```python
from build123d import *

# Parameters (mm, degrees)
MAIN_SHAPE_DEPTH        = 0.6
TABS_DEPTH              = 154.060061459
TABS_DEPTH_BACK         = 154.060061459
CHIN_GUARD_DEPTH        = 0.6
FILLET1_R               = 30
SKETCH8_W               = 100
SKETCH8_H               = 1
CUT_EXTRUDE3_DEPTH      = 0.2
BOSS_EXTRUDE1_START     = -0.6
BOSS_EXTRUDE1_DEPTH     = 0.6
CUT_EXTRUDE4_DEPTH      = 173.475044334
CUT_EXTRUDE4_DEPTH_BACK = 173.475044334
FILLET2_R               = 0.5
FILLET3_R               = 1.5


with BuildPart() as part:
    # Sketch1 → Main Shape (new body)
    with BuildSketch(Plane.XY):
        with BuildLine():
            Line((-24, -91.764766734), (24, -91.764766734))
            Line((24, -91.764766734), (78.266232563, -84.05670244))
            ThreePointArc((78.266232563, -84.05670244), (97.655491519, -79.289252293), (115.711102551, -70.764766734))
            ThreePointArc((115.711102551, -70.764766734), (120.685143325, -65.658407438), (122.5, -58.764766734))
            ThreePointArc((122.5, -58.764766734), (120.227482046, -43.118277124), (113.597722286, -28.764766734))
            ThreePointArc((113.597722286, -28.764766734), (107.811505455, -22.955172168), (100.180351554, -19.955641477))
            Line((100.180351554, -19.955641477), (60.74391922, -13.264766734))
            ThreePointArc((60.74391922, -13.264766734), (50.804108255, -9.246591688), (43.461443341, -1.434367632))
            ThreePointArc((43.461443341, -1.434367632), (36.448172688, 5.805997675), (26.941855461, 9.15842781))
            Line((26.941855461, 9.15842781), (17, 10.235233266))
            Line((17, 10.235233266), (10, 0))
            Line((10, 0), (-10, 0))
            Line((-10, 0), (-17, 10.235233266))
            Line((-17, 10.235233266), (-26.941855461, 9.15842781))
            ThreePointArc((-26.941855461, 9.15842781), (-36.448172688, 5.805997675), (-43.461443341, -1.434367632))
            ThreePointArc((-43.461443341, -1.434367632), (-50.804108255, -9.246591688), (-60.74391922, -13.264766734))
            Line((-60.74391922, -13.264766734), (-100.180351554, -19.955641477))
            ThreePointArc((-100.180351554, -19.955641477), (-107.811505455, -22.955172168), (-113.597722286, -28.764766734))
            ThreePointArc((-113.597722286, -28.764766734), (-120.227482046, -43.118277124), (-122.5, -58.764766734))
            ThreePointArc((-122.5, -58.764766734), (-120.685143325, -65.658407438), (-115.711102551, -70.764766734))
            ThreePointArc((-115.711102551, -70.764766734), (-97.655491519, -79.289252293), (-78.266232563, -84.05670244))
            Line((-78.266232563, -84.05670244), (-24, -91.764766734))
        make_face()
    extrude(amount=MAIN_SHAPE_DEPTH)

    # Sketch2 → Tabs (cut, two sides: drawn at the far end of the back side and taken through both)
    with BuildSketch(Plane.XY.offset(0.6).offset(-TABS_DEPTH_BACK)):
        with BuildLine():
            Line((-121.15, -59.764766734), (-121.15, -57.764766734))
            Line((-121.15, -57.764766734), (-115.985504489, -54.767473344))
            ThreePointArc((-115.985504489, -54.767473344), (-113.65344245, -43.380285918), (-108.686779625, -32.871298753))
            Line((-108.686779625, -32.871298753), (-111.02, -27.374766734))
            Line((-111.02, -27.374766734), (-109.82, -25.774766734))
            Line((-109.82, -25.774766734), (-107.82, -24.774766734))
            Line((-107.82, -24.774766734), (-106.22, -25.974766734))
            Line((-106.22, -25.974766734), (-107.42, -27.574766734))
            Line((-107.42, -27.574766734), (-105.82, -28.774766734))
            Line((-105.82, -28.774766734), (-99.063546264, -19.766161753))
            Line((-99.063546264, -19.766161753), (-100.180351554, -19.955641477))
            ThreePointArc((-100.180351554, -19.955641477), (-107.811505455, -22.955172168), (-113.597722286, -28.764766734))
            ThreePointArc((-113.597722286, -28.764766734), (-120.227482046, -43.118277124), (-122.5, -58.764766734))
            ThreePointArc((-122.5, -58.764766734), (-120.810564569, -65.431850055), (-116.15, -70.489846692))
            Line((-116.15, -70.489846692), (-116.15, -59.764766734))
            Line((-116.15, -59.764766734), (-118.15, -59.764766734))
            Line((-118.15, -59.764766734), (-118.15, -61.764766734))
            Line((-118.15, -61.764766734), (-120.15, -61.764766734))
            Line((-120.15, -61.764766734), (-121.15, -59.764766734))
        make_face()
        with BuildLine():
            Line((105.82, -28.774766734), (99.063546264, -19.766161753))
            Line((99.063546264, -19.766161753), (100.180351554, -19.955641477))
            ThreePointArc((100.180351554, -19.955641477), (107.811505455, -22.955172168), (113.597722286, -28.764766734))
            ThreePointArc((113.597722286, -28.764766734), (120.227482046, -43.118277124), (122.5, -58.764766734))
            ThreePointArc((122.5, -58.764766734), (120.810564569, -65.431850055), (116.15, -70.489846692))
            Line((116.15, -70.489846692), (116.15, -59.764766734))
            Line((116.15, -59.764766734), (118.15, -59.764766734))
            Line((118.15, -59.764766734), (118.15, -61.764766734))
            Line((118.15, -61.764766734), (120.15, -61.764766734))
            Line((120.15, -61.764766734), (121.15, -59.764766734))
            Line((121.15, -59.764766734), (121.15, -57.764766734))
            Line((121.15, -57.764766734), (115.985504489, -54.767473344))
            ThreePointArc((115.985504489, -54.767473344), (113.65344245, -43.380285918), (108.686779625, -32.871298753))
            Line((108.686779625, -32.871298753), (111.02, -27.374766734))
            Line((111.02, -27.374766734), (109.82, -25.774766734))
            Line((109.82, -25.774766734), (107.82, -24.774766734))
            Line((107.82, -24.774766734), (106.22, -25.974766734))
            Line((106.22, -25.974766734), (107.42, -27.574766734))
            Line((107.42, -27.574766734), (105.82, -28.774766734))
        make_face()
    extrude(amount=TABS_DEPTH + TABS_DEPTH_BACK, mode=Mode.SUBTRACT)

    # Sketch5 → Chin guard (add)
    with BuildSketch(Plane.XY.offset(0.6)):
        Polygon((-78.266232563, -84.05670244), (-24, -121.764766734), (24, -121.764766734), (78.266232563, -84.05670244), (24, -91.764766734), (-24, -91.764766734), align=None)
    extrude(amount=-CHIN_GUARD_DEPTH)

    # Fillet1
    fillet1_edges = [part.edges().sort_by_distance(p)[0] for p in [
        (-24, -121.764766734, 0.3),
        (24, -121.764766734, 0.3),
        (78.266232563, -84.05670244, 0.3),
        (-78.266232563, -84.05670244, 0.3),
    ]]
    fillet(fillet1_edges, radius=FILLET1_R)

    # Sketch8 → Cut-Extrude3 (cut)
    with BuildSketch(Plane.XY.offset(0.6)):
        with Locations((0, -4.5)):
            Rectangle(SKETCH8_W, SKETCH8_H)
    extrude(amount=-CUT_EXTRUDE3_DEPTH, mode=Mode.SUBTRACT)

    # Sketch9 → Boss-Extrude1 (add)
    with BuildSketch(Plane.XY.offset(0.6).offset(BOSS_EXTRUDE1_START)):
        with BuildLine():
            Line((-121.15, -61.764766734), (-120.15, -61.764766734))
            Line((-120.15, -61.764766734), (-121.15, -59.764766734))
            Line((-121.15, -59.764766734), (-121.15, -57.764766734))
            Line((-121.15, -57.764766734), (-115.985504489, -54.767473344))
            ThreePointArc((-115.985504489, -54.767473344), (-115.959300984, -54.461436848), (-115.931165822, -54.155571889))
            Line((-115.931165822, -54.155571889), (-122.15, -57.764766734))
            Line((-122.15, -57.764766734), (-122.15, -59.764766734))
            Line((-122.15, -59.764766734), (-121.15, -61.764766734))
        make_face()
        with BuildLine():
            Line((-111.02, -27.374766734), (-108.686779625, -32.871298753))
            ThreePointArc((-108.686779625, -32.871298753), (-108.849438719, -33.131850053), (-109.010449565, -33.393423117))
            Line((-109.010449565, -33.393423117), (-111.82, -26.774766734))
            Line((-111.82, -26.774766734), (-110.62, -25.174766734))
            Line((-110.62, -25.174766734), (-108.62, -24.174766734))
            Line((-108.62, -24.174766734), (-107.82, -24.774766734))
            Line((-107.82, -24.774766734), (-109.82, -25.774766734))
            Line((-109.82, -25.774766734), (-111.02, -27.374766734))
        make_face()
        with BuildLine():
            Line((108.62, -24.174766734), (107.82, -24.774766734))
            Line((107.82, -24.774766734), (109.82, -25.774766734))
            Line((109.82, -25.774766734), (111.02, -27.374766734))
            Line((111.02, -27.374766734), (108.686779625, -32.871298753))
            ThreePointArc((108.686779625, -32.871298753), (108.849438719, -33.131850053), (109.010449565, -33.393423117))
            Line((109.010449565, -33.393423117), (111.82, -26.774766734))
            Line((111.82, -26.774766734), (110.62, -25.174766734))
            Line((110.62, -25.174766734), (108.62, -24.174766734))
        make_face()
        with BuildLine():
            Line((121.15, -57.764766734), (115.985504489, -54.767473344))
            ThreePointArc((115.985504489, -54.767473344), (115.959300984, -54.461436848), (115.931165822, -54.155571889))
            Line((115.931165822, -54.155571889), (122.15, -57.764766734))
            Line((122.15, -57.764766734), (122.15, -59.764766734))
            Line((122.15, -59.764766734), (121.15, -61.764766734))
            Line((121.15, -61.764766734), (120.15, -61.764766734))
            Line((120.15, -61.764766734), (121.15, -59.764766734))
            Line((121.15, -59.764766734), (121.15, -57.764766734))
        make_face()
    extrude(amount=BOSS_EXTRUDE1_DEPTH)

    # Sketch7 → Cut-Extrude4 (cut, two sides: drawn at the far end of the back side and taken through both)
    with BuildSketch(Plane.XY.offset(0.6).offset(-CUT_EXTRUDE4_DEPTH_BACK)):
        with BuildLine():
            Line((-103.838644773, -41.913383247), (-112.792739682, -41.005537243))
            ThreePointArc((-112.792739682, -41.005537243), (-111.068159087, -37.116718005), (-109.010449565, -33.393423117))
            Line((-109.010449565, -33.393423117), (-102.436901217, -38.323584378))
            ThreePointArc((-102.436901217, -38.323584378), (-101.773894786, -40.651050555), (-103.838644773, -41.913383247))
        make_face()
        with BuildLine():
            Line((109.010449565, -33.393423117), (102.436901217, -38.323584378))
            ThreePointArc((102.436901217, -38.323584378), (101.773894786, -40.651050555), (103.838644773, -41.913383247))
            Line((103.838644773, -41.913383247), (112.792739682, -41.005537243))
            ThreePointArc((112.792739682, -41.005537243), (111.068159087, -37.116718005), (109.010449565, -33.393423117))
        make_face()
    extrude(amount=CUT_EXTRUDE4_DEPTH + CUT_EXTRUDE4_DEPTH_BACK, mode=Mode.SUBTRACT)

    # Fillet2
    fillet2_edges = [part.edges().sort_by_distance(p)[0] for p in [
        (109.010449565, -33.393423117, 0.3),
        (-112.792739682, -41.005537243, 0.3),
        (-109.010449565, -33.393423117, 0.3),
        (-106.22, -25.974766734, 0.3),
        (-107.42, -27.574766734, 0.3),
        (-105.82, -28.774766734, 0.3),
        (-115.931165822, -54.155571889, 0.3),
        (-118.15, -61.764766734, 0.3),
        (-116.15, -59.764766734, 0.3),
        (-118.15, -59.764766734, 0.3),
        (118.15, -61.764766734, 0.3),
        (118.15, -59.764766734, 0.3),
        (116.15, -59.764766734, 0.3),
        (105.82, -28.774766734, 0.3),
        (107.42, -27.574766734, 0.3),
        (106.22, -25.974766734, 0.3),
        (116.15, -70.489846692, 0.3),
        (115.931165822, -54.155571889, 0.3),
        (112.792739682, -41.005537243, 0.3),
        (99.063546264, -19.766161753, 0.3),
        (-99.063546264, -19.766161753, 0.3),
        (-116.15, -70.489846692, 0.3),
    ]]
    fillet(fillet2_edges, radius=FILLET2_R)

    # Fillet3
    fillet3_edges = [part.edges().sort_by_distance(p)[0] for p in [
        (-122.15, -57.764766734, 0.3),
        (-122.15, -59.764766734, 0.3),
        (-121.15, -61.764766734, 0.3),
        (-108.62, -24.174766734, 0.3),
        (-110.62, -25.174766734, 0.3),
        (-111.82, -26.774766734, 0.3),
        (121.15, -61.764766734, 0.3),
        (122.15, -59.764766734, 0.3),
        (122.15, -57.764766734, 0.3),
        (111.82, -26.774766734, 0.3),
        (110.62, -25.174766734, 0.3),
        (108.62, -24.174766734, 0.3),
    ]]
    fillet(fillet3_edges, radius=FILLET3_R)


solid = part.part
```
Input: part model. Units: mm. Frame: model coordinates. A direction names the side the tool comes from. Coordinates: 2 decimals unless noted, no trailing zeros. Order: outer loops, then holes, each group sorted by start corner. A loop starts at its lowest first (then second) coordinate and runs counter-clockwise, first axis right, second up. Notation, with made-up numbers: (43, -13) - (48, -13) arc R14 ccw to (48, 6) - close; hole circle Ø6 at (-5, 46.25). An arc over 180 degrees is marked (long way). Put each result on its own line as item: value.
1. Cut plane B-B on y = -104.5. Return the cut outline in (x, z), then the cut area to 3 significant figures.
Report:
outline: (-48.85, 0) - (48.85, 0) - (48.85, 0.6) - (-48.85, 0.6) - close
area: 58.6 mm2
2. Reachability of faces 1 (the face through (102.396, -24.209, 0.296)), 2 (the face through (-2, -63, 0.6)) from +Z, -Z, +X, -X, +Y, -Y: full face, straight path, thin tool, end or side. Return the list, or none.
Report:
face 1: +Z, -Z, +Y
face 2: +Z, +X, -X, +Y, -Y
3. Draft query along Y for faces 3 (the face through (-105.72, -35.86, 0.3)), 4 (the face through (-78.087, -84.918, 0.304)), 5 (the face through (105.72, -35.86, 0.3)), 6 (the face through (-102.396, -24.209, 0.296)). Return one class per face: pulls with the +Y half, pulls with the -Y half, needs draft (parallel to the pull), parting line crosses it, or undercut.
Report:
face 3: undercut
face 4: pulls with the -Y half
face 5: undercut
face 6: pulls with the +Y half
4. Line query: line 1 along X through (y, z) = (-75, 0.3); line 2 along Y through (x, z) = (-1.5, 0.2); line 3 along X through (y, z) = (2.5, 0.45). Output: solid intervals per line, ascending.
Report:
line 1: x = -107.9 to 107.9
line 2: y = -121.76 to 0
line 3: x = -40.46 to -11.71, 11.71 to 40.46
5. Cut plane A-A on x = 76.5. Return the cut outline in (y, z).
Report:
outline: (-85.66, 0) - (-15.94, 0) - (-15.94, 0.6) - (-85.66, 0.6) - close
6. Contact query for a flat-ended pin moving along its axis: pin 1 Ø0.8 at (x, y) = (6.5, -4.5) entering from +Z. Output: stop coordinate, or through.
Report:
pin 1: stops at z = 0.4
